Design review of the part built by this model. Coordinates are the model's own, in mm. A direction names the side the tool comes from. Round coordinates to 2 decimals unless told otherwise and drop trailing zeros. Loops run counter-clockwise (first coordinate to the right, second up) from the corner with the lowest first, then second, coordinate; pieces in that order, holes last. Notation, with made-up numbers: (25, 76) - (58, 76) arc R23 ccw to (58, 86) - close; hole circle Ø6 at (1.25, 43.25). An arc over 180 degrees is marked (long way). Answer as CSV lines item,"result". Start each with the question number.
(1) For P1, Ø4.5, axis at x = -23, y = 17.5, coming from the +Z side; P2, Ø5, axis at x = 18, y = 14.5, coming from the -Z side; P3, Ø1.5, axis at x = -11.5, y = 16.5, coming from the +Z side, all flat-tipped, find the tip position at first contact; note any pin that passes through.
(2) Wall thickness on L1, parallel to X at y = 13.5, z = 0 (3 decimals); L2, parallel to Y at x = 23.5, z = -3.5; L3, parallel to X at y = 17.25, z = 20.5: over which ranges is each line inside the solid? List them lowest first.
(3) Consider section B-B (y = 11.5). Give the boundary of the cut face in (x, z) (3 decimals).
(4) For faces 1 (the flat face through (-26, 17, -1)), 2 (the cylindrical face through (19.524, 8.344, 4.336)), 3 (the flat face through (-17.5, 10, 10.1)), 4 (the cylindrical face through (2.15, 13.94, -1.12)), list the 3-axis set-ups (+Z, -Z, +X, -X, +Y, -Y) from which the entire face can be reached by the end or side of a thin tool; tool diameter is ignored.
(5) Consider section C-C (y = 5.75). Give the boundary of the cut face in (x, z), and give its area (3 significant figures).
(6) Mouldability with a two-part tool opening along Y and no side actions: class faces 5 (the cylindrical face through (-22.989, 17.797, -0.014)), 6 (the flat face through (17.5, 10, -10.1)), 7 (the cylindrical face through (-17.675, 5.809, -10.226)) as released by +Y, released by -Y, zero draft, split by the parting line, or undercut.
from build123d import *

# Parameters (mm, degrees)
BOSS_EXTRUDE1_START = -10
BOSS_EXTRUDE1_DEPTH = 10
CHAMFER1_SIZE       = 1
SKETCH4_W           = 3.87
SKETCH4_H           = 2
CUT_EXTRUDE1_DEPTH  = 44.920382512
FILLET1_R           = 4


with BuildPart() as part:
    # Sketch1 → Revolve1 (revolve)
    with BuildSketch(Plane.XY, mode=Mode.PRIVATE) as revolve1_sk:
        Polygon((0, 0), (20, 0), (20, 15), (28, 15), (28, 19), (2.425, 19), (2.425, 9), (0, 9), align=None)
    revolve(revolve1_sk.sketch.rotate(Axis((0, 0, 0), (0, 1, 0)), 90), axis=Axis((0, 0, 0), (0, 1, 0)))

    # Sketch2 → Boss-Extrude1 (add)
    with BuildSketch(Plane.XZ.offset(BOSS_EXTRUDE1_START)):
        with BuildLine():
            ThreePointArc((-1.25, 19.960899278), (0, 20.42), (1.25, 19.960899278))
            ThreePointArc((1.25, 19.960899278), (10, 17.320508076), (16.661645857, 11.062981394))
            ThreePointArc((16.661645857, 11.062981394), (17.684238745, 10.21), (17.911645857, 8.897917884))
            ThreePointArc((17.911645857, 8.897917884), (20, 0), (17.911645857, -8.897917884))
            ThreePointArc((17.911645857, -8.897917884), (17.684238745, -10.21), (16.661645857, -11.062981394))
            ThreePointArc((16.661645857, -11.062981394), (10, -17.320508076), (1.25, -19.960899278))
            ThreePointArc((1.25, -19.960899278), (0, -20.42), (-1.25, -19.960899278))
            ThreePointArc((-1.25, -19.960899278), (-10, -17.320508076), (-16.661645857, -11.062981394))
            ThreePointArc((-16.661645857, -11.062981394), (-17.684238745, -10.21), (-17.911645857, -8.897917884))
            ThreePointArc((-17.911645857, -8.897917884), (-20, 0), (-17.911645857, 8.897917884))
            ThreePointArc((-17.911645857, 8.897917884), (-17.684238745, 10.21), (-16.661645857, 11.062981394))
            ThreePointArc((-16.661645857, 11.062981394), (-10, 17.320508076), (-1.25, 19.960899278))
        make_face()
    extrude(amount=BOSS_EXTRUDE1_DEPTH)

    # Sketch3 → Cut-Revolve1 (revolve, cut)
    with BuildSketch(Plane.XY, mode=Mode.PRIVATE) as cut_revolve1_sk:
        Polygon((-21, 3.232050808), (-18.556624327, -1), (-21, -1), align=None)
    revolve(cut_revolve1_sk.sketch.rotate(Axis((0, 29.336873575, 0), (0, -1, 0)), 273.58332148), axis=Axis((0, 29.336873575, 0), (0, -1, 0)), mode=Mode.SUBTRACT)

    # Chamfer1
    chamfer1_edges = [part.edges().sort_by_distance(p)[0] for p in [
        (0, 19, 2.425),
        (0, 19, 28),
        (0, 15, 28),
    ]]
    chamfer(chamfer1_edges, length=CHAMFER1_SIZE)

    # Sketch4 → Cut-Extrude1 (cut, through all)
    with BuildSketch(Plane.XZ):
        with Locations((-26.065, 0)):
            Rectangle(SKETCH4_W, SKETCH4_H)
    extrude(amount=-CUT_EXTRUDE1_DEPTH, mode=Mode.SUBTRACT)

    # Fillet1
    fillet1_edges = [part.edges().sort_by_distance(p)[0] for p in [
        (-24.13, 19, 0),
    ]]
    fillet(fillet1_edges, radius=FILLET1_R - 0.0001)  # a hair under: the kernel refuses the full size


solid = part.part
Determined:
1,P1,"stops at z = 18.8"
1,P2,"stops at z = -22.98"
1,P3,"stops at z = 25.85"
2,L1,"x = -20 to -2.425, 2.425 to 20"
2,L2,"y = 15 to 19"
2,L3,"x = -19.07 to 19.07"
3,outline,"circle Ø40 at (0, 0); hole circle Ø4.85 at (0, 0)"
4,face 1,"-X, +Y"
4,face 2,"none"
4,face 3,"+Z, -X"
4,face 4,"+Y"
5,outline,"(-17.91, -8.9) arc R1.93 ccw to (-16.66, -11.06) arc R20 ccw to (-1.25, -19.96) arc R1.93 ccw to (1.25, -19.96) arc R20 ccw to (16.66, -11.06) arc R1.93 ccw to (17.91, -8.9) arc R20 ccw to (17.91, 8.9) arc R1.93 ccw to (16.66, 11.06) arc R20 ccw to (1.25, 19.96) arc R1.93 ccw to (-1.25, 19.96) arc R20 ccw to (-16.66, 11.06) arc R1.93 ccw to (-17.91, 8.9) arc R20 ccw to start"
5,area,"1,260 mm^2"
6,face 5,"released by +Y"
6,face 6,"undercut"
6,face 7,"zero draft"
